Source: CAD feature listing. Evaluate the final solid. Frame: model axes, mm. A direction names the side the tool comes from. Give positions to 0.01 mm unless a question says otherwise; leave off trailing zeros. Write each loop counter-clockwise with the first axis right and the second up, starting at its lowest first coordinate (ties: lowest second). Pieces come first, ordered by that corner, then holes. Notation, with made-up numbers: (22.25, 9) - (59.25, 9) arc R18 ccw to (59.25, 20) - close; hole circle Ø5 at (25, -39). An arc over 180 degrees is marked (long way). Answer as a JSON object with one key per item and string values. Group by question number.
from build123d import *

# Parameters (mm, degrees)
SKETCH_1_R        = 1
EXTRUDE_198_DEPTH = 40
PH1_START         = 1.31
PH1_DEPTH         = 0.96


with BuildPart() as part:
    # 草图1 → Extrude 198 (new body)
    with BuildSketch(Plane.XY):
        Circle(SKETCH_1_R)
    extrude(amount=-EXTRUDE_198_DEPTH)

    # 草图6 → Revolve 324 (revolve)
    with BuildSketch(Plane(origin=(0, 0, 0), x_dir=(1, 0, 0), z_dir=(0, 1, 0)), mode=Mode.PRIVATE) as revolve_324_sk:
        with BuildLine():
            Line((0, 0), (1.75, 0))
            Line((1.75, 0), (1.75, -0.585357107))
            ThreePointArc((1.75, -0.585357107), (0.945147404, -1.114453798), (0, -1.3))
            Line((0, -1.3), (0, 0))
        make_face()
    revolve(revolve_324_sk.sketch.rotate(Axis((0, 0, -2), (0, 0, 1)), 180), axis=Axis((0, 0, -2), (0, 0, 1)))

    # 草图7 → 十字槽_PH1_简化 (cut)
    with BuildSketch(Plane.XY.offset(PH1_START)):
        Polygon((-0.3, -1.1), (0.3, -1.1), (0.3, -0.3), (1.1, -0.3), (1.1, 0.3), (0.3, 0.3), (0.3, 1.1), (-0.3, 1.1), (-0.3, 0.3), (-1.1, 0.3), (-1.1, -0.3), (-0.3, -0.3), align=None)
    extrude(amount=-PH1_DEPTH, mode=Mode.SUBTRACT)


solid = part.part
Q1. Ray query, probe 1 along Y at (x, z) = (-0.05, -34); probe 2 along X at (y, z) = (-0.1, -8); probe 3 along Z at (x, y) = (-0.2, 0.6). Return the intervals inside material, ascending. Write a range as [from, to].
Q2. Reachability of faces 1 (the flat face through (1, 1, 0)), 2 (the cylindrical face through (-1.617, 0.67, 0.297)), 3 (the flat face through (-0.3, -0.7, 0.8)) from +Z, -Z, +X, -X, +Y, -Y: full face, straight path, thin tool, end or side. Return the list, or none.
Q3. Section A-A on z = -9.5. Return the cut outline in (x, y), then the cut area to 3 significant figures.
Q4. Draft query along X for faces 4 (the flat face through (0.3, 0.7, 0.8)), 5 (the cylindrical face through (0, -1, -20)), 6 (the flat face through (0, 0, -40)). Return one class per face: released by +X, released by -X, zero draft, split by the parting line, or undercut.
Q5. First-contact query: pin 1 Ø1.5 at (x, z) = (-1, -29.5) entering from -Y; pin 2 Ø0.6 at (x, z) = (-0.5, 1) entering from -Y; pin 3 Ø1.5 at (y, z) = (0, -31.5) entering from -X; pin 4 Ø2 at (x, y) = (1, -1.5) entering from -Z. Flat tips, straight axial feed; report the tip coordinate or a pass-through.
Taken from the geometry:
{
 "1": {"probe 1": "y = [-1, 1]", "probe 2": "x = [-0.99, 0.99]", "probe 3": "z = [-40, 0.35]"},
 "2": {"face 1": "-Z", "face 2": "+Z, -Z", "face 3": "+Z"},
 "3": {"outline": "circle Ø2 at (0, 0)", "area": "3.14 mm²"},
 "4": {"face 4": "undercut", "face 5": "split by the parting line", "face 6": "zero draft"},
 "5": {"pin 1": "stops at y = -0.97", "pin 2": "stops at y = -1.56", "pin 3": "stops at x = -1", "pin 4": "stops at z = -40"}
}
